from build123d import *

# Parameters (mm, degrees)
SKETCH1_R           = 5
BOSS_EXTRUDE2_DEPTH = 40
CHAMFER1_SIZE       = 5


with BuildPart() as part:
    # Sketch1 → Boss-Extrude2 (new body)
    with BuildSketch(Plane(origin=(0, 0, 0), x_dir=(1, 0, 0), z_dir=(0, 1, 0))):
        with BuildLine():
            Line((-60, 60), (-34.43523791, 60))
            Line((-34.43523791, 60), (-29.43523791, 55))
            Line((-29.43523791, 55), (-29.43523791, 40))
            Line((-29.43523791, 40), (-24.43523791, 35))
            Line((-24.43523791, 35), (24.43523791, 35))
            Line((24.43523791, 35), (29.43523791, 40))
            Line((29.43523791, 40), (29.43523791, 55))
            Line((29.43523791, 55), (34.43523791, 60))
            Line((34.43523791, 60), (60, 60))
            ThreePointArc((60, 60), (67.071067812, 57.071067812), (70, 50))
            Line((70, 50), (70, -50))
            ThreePointArc((70, -50), (67.071067812, -57.071067812), (60, -60))
            Line((60, -60), (-60, -60))
            ThreePointArc((-60, -60), (-67.071067812, -57.071067812), (-70, -50))
            Line((-70, -50), (-70, 50))
            ThreePointArc((-70, 50), (-67.071067812, 57.071067812), (-60, 60))
        make_face()
        with Locations((-60, 50)):
            Circle(SKETCH1_R, mode=Mode.SUBTRACT)
        with Locations((60, 50)):
            Circle(SKETCH1_R, mode=Mode.SUBTRACT)
        with Locations((60, -50)):
            Circle(SKETCH1_R, mode=Mode.SUBTRACT)
        with Locations((-60, -50)):
            Circle(SKETCH1_R, mode=Mode.SUBTRACT)
        with BuildLine():
            Line((-40, 10), (40, 10))
            ThreePointArc((40, 10), (50, 0), (40, -10))
            Line((40, -10), (-40, -10))
            ThreePointArc((-40, -10), (-50, 0), (-40, 10))
        make_face(mode=Mode.SUBTRACT)
    extrude(amount=BOSS_EXTRUDE2_DEPTH)

    # Chamfer1
    chamfer1_edges = [part.edges().sort_by_distance(p)[0] for p in [
        (-50, 0, 0),
        (0, 0, 10),
        (50, 0, 0),
        (0, 0, -10),
        (-50, 40, 0),
        (0, 40, 10),
        (50, 40, 0),
        (0, 40, -10),
    ]]
    chamfer(chamfer1_edges, length=CHAMFER1_SIZE)


solid = part.part
The listing builds one solid part. Answer for the finished solid, in the listing's coordinates (mm). A direction names the side the tool comes from. Round coordinates to 2 decimals unless told otherwise and drop trailing zeros. Write each loop counter-clockwise with the first axis right and the second up, starting at its lowest first coordinate (ties: lowest second). Pieces come first, ordered by that corner, then holes. Notation, with made-up numbers: (25.25, 70.5) - (50.25, 70.5) arc R33 cw to (50.25, 102.5) - close; hole circle Ø6 at (-4.5, 20). An arc over 180 degrees is marked (long way). Use a Markdown table: item, result. Add a question column.
1. A flat-ended cylindrical pin translates along its axis: P1, Ø24, axis at x = 11, y = 24.5, coming from the -Z side. Find the tip coordinate at first contact, or state that the pin passes through.
2. The part is cut by section A-A (z = 0). Write down the section's boundary in (x, y).
3. For a pull along X with two mould halves and no side action, classify faces 5 (the face through (66.99, 19.72, -57.15)), 6 (the face through (0, 20, -35)), 7 (the face through (1, 40, 26)) as +X half, -X half, draft (parallel to the pull), parting line (faces both ways), or undercut.
4. A tool of negligible diameter and unlimited length cuts with its end or side. For faces 1 (the face through (-29.435, 20, -48)), 2 (the face through (1, 2, 13)), 3 (the face through (1, 20, 10)), 4 (the face through (50.3, 35.3, -0.2)), from which of +Z, -Z, +X, -X, +Y, -Y can it reach the whole face along a straight path? Write none if from no direction.
5. Consider line 1 (X direction, y = 11, z = 50); line 2 (Z direction, x = -60, y = 11); line 3 (Z direction, x = -37, y = 15). Determine where each line is inside the solid, lowest interval first.
6. The part is cut by section B-B (x = -5). Write down the section's boundary in (y, z), and give its area (3 significant figures).
7. The part is cut by section C-C (y = 19.5). Write down the section's boundary in (x, z), and give its area (3 significant figures).
Reported:
| question | item | result |
|---|---|---|
| 1 | P1 | z = -35 |
| 2 | outline | (-70, 0) - (-55, 0) - (-50, 5) - (-50, 35) - (-55, 40) - (-70, 40) - close; (50, 5) - (55, 0) - (70, 0) - (70, 40) - (55, 40) - (50, 35) - close |
| 3 | face 5 | +X half |
| 3 | face 6 | undercut |
| 3 | face 7 | draft |
| 4 | face 1 | -Z, +Y, -Y |
| 4 | face 2 | -Y |
| 4 | face 3 | +Y, -Y |
| 4 | face 4 | +Y |
| 5 | line 1 | -70 to -65, -55 to 55, 65 to 70 |
| 5 | line 2 | -60 to -55, -45 to 45, 55 to 60 |
| 5 | line 3 | -60 to -10, 10 to 60 |
| 6 | outline | (0, -35) - (40, -35) - (40, -15) - (35, -10) - (5, -10) - (0, -15) - close; (0, 15) - (5, 10) - (35, 10) - (40, 15) - (40, 60) - (0, 60) - close |
| 6 | area | 2,950 mm^2 |
| 7 | outline | (-70, -50) arc R10 ccw to (-60, -60) - (-34.44, -60) - (-29.44, -55) - (-29.44, -40) - (-24.44, -35) - (24.44, -35) - (29.44, -40) - (29.44, -55) - (34.44, -60) - (60, -60) arc R10 ccw to (70, -50) - (70, 50) arc R10 ccw to (60, 60) - (-60, 60) arc R10 ccw to (-70, 50) - close; hole circle Ø10 at (-60, -50); hole circle Ø10 at (-60, 50); hole (-40, -10) - (40, -10) arc R10 ccw to (40, 10) - (-40, 10) arc R10 ccw to start; hole circle Ø10 at (60, -50); hole circle Ø10 at (60, 50) |
| 7 | area | 13,000 mm^2 |
